from build123d import *

# Parameters (mm, degrees)
F0_R     = 47.5522600406
F1_DEPTH = 10
F2_R     = 5
F3_R     = 4.99999


# Not quite as in the source:
# - a fillet or chamfer is up to 0.001 mm smaller than in the source, because OpenCascade refuses the exact size


with BuildPart() as f1:
    # F0 (on Top) → F1 (new body)
    with BuildSketch(Plane.XY):
        Circle(F0_R)
    extrude(amount=F1_DEPTH)

    # F2
    f2_edges = [f1.edges().sort_by_distance(p)[0] for p in [
        (-47.55226, 0, 10),
    ]]
    fillet(f2_edges, radius=F2_R)

    # F3 (radius 5 in the source; OpenCascade refuses exactly that, so slightly less here)
    f3_edges = [f1.edges().sort_by_distance(p)[0] for p in [
        (-47.55226, 0, 0),
    ]]
    fillet(f3_edges, radius=F3_R)


solid = f1.part
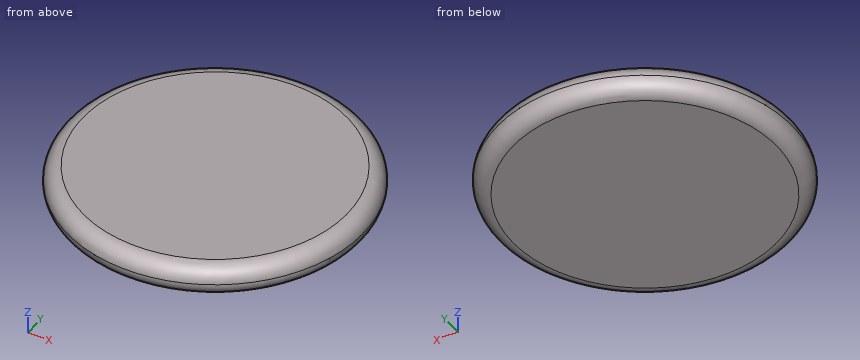
Part model, mm, in its own coordinate system. Coordinates: 2 decimals unless noted, no trailing zeros. Write each loop counter-clockwise with the first axis right and the second up, starting at its lowest first coordinate (ties: lowest second). Pieces come first, ordered by that corner, then holes. Notation, with made-up numbers: M 11,65.25 L 15,65.25 A21 ccw 15,101.25 Z; hole C -26.5,58 d7. An arc over 180 degrees is marked long. Return JSON: item names as keys, results as strings.
1. Flat gauge pins, fed straight in: pin 1 Ø3 at (x, z) = (-28.5, 7.5) entering from +Y; pin 2 Ø6 at (y, z) = (-24.5, 4) entering from +X; pin 3 Ø1 at (x, z) = (7.5, 8) entering from +Y. Where does each tip first touch, or does it go through?
Determined:
{"pin 1": "y = 38.62", "pin 2": "x = 42.37", "pin 3": "y = 46.29"}
2. Probe L1, parallel to X at y = 9, z = 9.5; L2, parallel to X at y = -15, z = 9; L3, parallel to Y at x = -39, z = 4.75. List the from-to ranges inside material, lowest first.
Determined:
{"L1": "-43.82 to 43.82", "L2": "-43.01 to 43.01", "L3": "-27.2 to 27.2"}
3. Saw through at C-C, the plane z = 3.25. Write the cut outline in (x, y), then the cut area to 3 significant figures.
Determined:
{"outline": "C 0,0 d94.47", "area": "7,010 mm²"}
